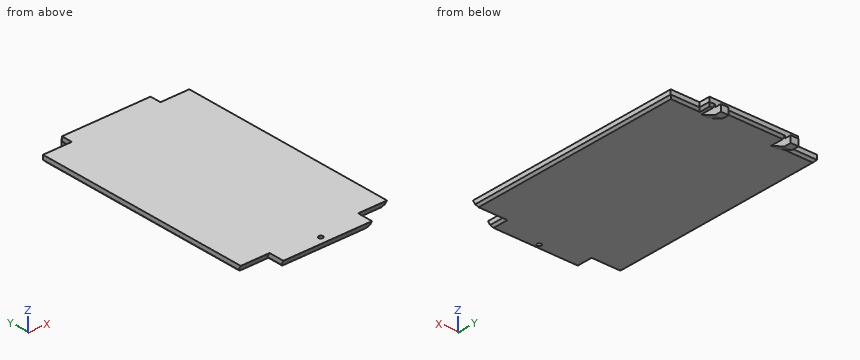
from build123d import *
from OCP.BRepFilletAPI import BRepFilletAPI_MakeChamfer

# Parameters (mm, degrees)
SKETCH_1_W          = 40
SKETCH_1_H          = 112
EXTRUDE_1_DEPTH     = 3
SKETCH_2_R          = 1
CUT_EXTRUDE_1_DEPTH = 3
SKETCH_3_W          = 3.5
SKETCH_3_H          = 10
EXTRUDE_2_DEPTH     = 3.2
CHAMFER_1_SIZE      = 6.8
CHAMFER_1_SIZE2     = 3.170892075
SKETCH_4_W          = 66
SKETCH_4_H          = 100
EXTRUDE_3_DEPTH     = 3
SKETCH_5_W          = 42.259647881
SKETCH_5_H          = 3.16572893
CUT_EXTRUDE_2_DEPTH = 0.2
CHAMFER_3_SIZE      = 1
CHAMFER_4_SIZE      = 2.944486373
CHAMFER_4_SIZE_2    = 1.7


with BuildPart() as part:
    # 草圖1 → 填料-伸長1 (new body)
    with BuildSketch(Plane.XY):
        with Locations((20, 56)):
            Rectangle(SKETCH_1_W, SKETCH_1_H)
    extrude(amount=EXTRUDE_1_DEPTH)

    # 草圖2 → 除料-伸長1 (cut)
    with BuildSketch(Plane.XY):
        with Locations((20, 3.5)):
            Circle(SKETCH_2_R)
    extrude(amount=CUT_EXTRUDE_1_DEPTH, mode=Mode.SUBTRACT)

    # 草圖3 → 填料-伸長2 (add)
    with BuildSketch(Plane.XY):
        with Locations((35.75, 110)):
            Rectangle(SKETCH_3_W, SKETCH_3_H)
        with Locations((4.25, 110)):
            Rectangle(SKETCH_3_W, SKETCH_3_H)
    extrude(amount=-EXTRUDE_2_DEPTH)

    # 導角1: one chamfer whose edges measure the first distance from different faces: ONE call of the kernel's chamfer builder (chamfer() names one face for all edges)
    chamfer_1_edges_1 = [part.edges().sort_by_distance(p)[0] for p in [
        (35.75, 105, -3.2),
    ]]
    chamfer_1_side_1 = [part.faces().sort_by_distance(p)[0] for p in [
        (35.75, 110, -3.2),
    ]]
    chamfer_1_edges_2 = [part.edges().sort_by_distance(p)[0] for p in [
        (4.25, 105, -3.2),
    ]]
    chamfer_1_side_2 = [part.faces().sort_by_distance(p)[0] for p in [
        (4.25, 110, -3.2),
    ]]
    chamfer_1 = BRepFilletAPI_MakeChamfer(part.part.solid().wrapped)
    for e in chamfer_1_edges_1:
        chamfer_1.Add(CHAMFER_1_SIZE, CHAMFER_1_SIZE2, e.wrapped, chamfer_1_side_1[0].wrapped)  # the first distance lies on this face
    for e in chamfer_1_edges_2:
        chamfer_1.Add(CHAMFER_1_SIZE, CHAMFER_1_SIZE2, e.wrapped, chamfer_1_side_2[0].wrapped)  # the first distance lies on this face
    add(Compound.cast(chamfer_1.Shape()), mode=Mode.REPLACE)

    # 草圖4 → 填料-伸長3 (add)
    with BuildSketch(Plane.XY):
        with Locations((20, 57)):
            Rectangle(SKETCH_4_W, SKETCH_4_H)
    extrude(amount=EXTRUDE_3_DEPTH)

    # 草圖5 → 除料-伸長2 (cut)
    with BuildSketch(Plane.XY):
        with Locations((18.12982394, 113.582864465)):
            Rectangle(SKETCH_5_W, SKETCH_5_H)
    extrude(amount=-CUT_EXTRUDE_2_DEPTH, mode=Mode.SUBTRACT)

    # 導角3
    chamfer_3_edges = [part.edges().sort_by_distance(p)[0] for p in [
        (20, 112, 0),
        (1.25, 112, 0),
        (38.75, 112, 0),
        (40, 3.5, 0),
        (0, 109.5, 0),
        (40, 109.5, 0),
        (0, 3.5, 0),
        (-6.5, 107, 0),
        (46.5, 107, 0),
        (53, 57, 0),
        (-13, 57, 0),
    ]]
    chamfer(chamfer_3_edges, length=CHAMFER_3_SIZE)

    # 導角4
    # the kernel refuses this chamfer: 2.944486373, 1.7 mm, written as the material it takes off along each edge
    with BuildSketch(Plane(origin=(8.61763875, 7, 0), x_dir=(0, -0.01932676561270069, 0.9998132206222079), z_dir=(-1, 0, 0))) as chamfer_4_piece_1_section:
        Polygon((CHAMFER_4_SIZE * 0.999813220577, CHAMFER_4_SIZE * 0.0193267656118), (-CHAMFER_4_SIZE_2 * 0.0193267656127, CHAMFER_4_SIZE_2 * 0.999813220622), (0, 0), align=None)
    chamfer_4_piece_1 = extrude(amount=28.2352775, mode=Mode.PRIVATE)
    chamfer_4_piece_1 = split(chamfer_4_piece_1, bisect_by=Plane(origin=(0.556062959, 7.780962214, 0.443937041), z_dir=(-0.7071067811865476, 0, -0.7071067811865476)), keep=Keep.TOP, mode=Mode.PRIVATE)
    chamfer_4_piece_1 = split(chamfer_4_piece_1, bisect_by=Plane(origin=(0, 7.780962214, 0.258582722), z_dir=(1, 0, 0)), keep=Keep.TOP, mode=Mode.PRIVATE)
    add(chamfer_4_piece_1, mode=Mode.SUBTRACT)
    with BuildSketch(Plane(origin=(8.61763875, 7, 0), x_dir=(0, -0.01932676561270069, 0.9998132206222079), z_dir=(-1, 0, 0))) as chamfer_4_piece_2_section:
        Polygon((CHAMFER_4_SIZE * 0.999813220577, CHAMFER_4_SIZE * 0.0193267656118), (-CHAMFER_4_SIZE_2 * 0.0193267656127, CHAMFER_4_SIZE_2 * 0.999813220622), (0, 0), align=None)
    chamfer_4_piece_2 = extrude(amount=28.2352775, mode=Mode.PRIVATE)
    chamfer_4_piece_2 = split(chamfer_4_piece_2, bisect_by=Plane(origin=(-0.79990122, 7.215436489, 1.79990122), z_dir=(0.7071067811865476, 0, 0.7071067811865476)), keep=Keep.TOP, mode=Mode.PRIVATE)
    chamfer_4_piece_2 = split(chamfer_4_piece_2, bisect_by=Plane(origin=(0, 7.215436489, 2.06653496), z_dir=(-1, 0, 0)), keep=Keep.TOP, mode=Mode.PRIVATE)
    add(chamfer_4_piece_2, mode=Mode.SUBTRACT)
    with BuildSketch(Plane(origin=(8.61763875, 7, 0), x_dir=(0, -0.01932676561270069, 0.9998132206222079), z_dir=(-1, 0, 0))) as chamfer_4_piece_3_section:
        Polygon((CHAMFER_4_SIZE * 0.999813220577, CHAMFER_4_SIZE * 0.0193267656118), (-CHAMFER_4_SIZE_2 * 0.0193267656127, CHAMFER_4_SIZE_2 * 0.999813220622), (0, 0), align=None)
    chamfer_4_piece_3 = extrude(amount=28.2352775, mode=Mode.PRIVATE)
    chamfer_4_piece_3 = split(chamfer_4_piece_3, bisect_by=Plane(origin=(-4.964199095, 7.550450485, 5.964199095), z_dir=(-0.7071067811865476, 0, -0.7071067811865476)), keep=Keep.TOP, mode=Mode.PRIVATE)
    chamfer_4_piece_3 = split(chamfer_4_piece_3, bisect_by=Plane(origin=(0, 7.550450485, 0.970145216), z_dir=(-1, 0, 0)), keep=Keep.TOP, mode=Mode.PRIVATE)
    add(chamfer_4_piece_3, mode=Mode.SUBTRACT)
    with BuildSketch(Plane(origin=(59.61763875, 7, 0), x_dir=(0, -0.01932676561270069, 0.9998132206222079), z_dir=(-1, 0, 0))) as chamfer_4_piece_4_section:
        Polygon((CHAMFER_4_SIZE * 0.999813220577, CHAMFER_4_SIZE * 0.0193267656118), (-CHAMFER_4_SIZE_2 * 0.0193267656127, CHAMFER_4_SIZE_2 * 0.999813220622), (0, 0), align=None)
    chamfer_4_piece_4 = extrude(amount=28.2352775, mode=Mode.PRIVATE)
    chamfer_4_piece_4 = split(chamfer_4_piece_4, bisect_by=Plane(origin=(40, 7.550450485, 0.970145216), z_dir=(1, 0, 0)), keep=Keep.TOP, mode=Mode.PRIVATE)
    chamfer_4_piece_4 = split(chamfer_4_piece_4, bisect_by=Plane(origin=(44.964199095, 7.550450485, 5.964199095), z_dir=(0.7071067811865476, 0, -0.7071067811865476)), keep=Keep.TOP, mode=Mode.PRIVATE)
    add(chamfer_4_piece_4, mode=Mode.SUBTRACT)
    with BuildSketch(Plane(origin=(59.61763875, 7, 0), x_dir=(0, -0.01932676561270069, 0.9998132206222079), z_dir=(-1, 0, 0))) as chamfer_4_piece_5_section:
        Polygon((CHAMFER_4_SIZE * 0.999813220577, CHAMFER_4_SIZE * 0.0193267656118), (-CHAMFER_4_SIZE_2 * 0.0193267656127, CHAMFER_4_SIZE_2 * 0.999813220622), (0, 0), align=None)
    chamfer_4_piece_5 = extrude(amount=28.2352775, mode=Mode.PRIVATE)
    chamfer_4_piece_5 = split(chamfer_4_piece_5, bisect_by=Plane(origin=(40, 7.780962214, 0.258582722), z_dir=(-1, 0, 0)), keep=Keep.TOP, mode=Mode.PRIVATE)
    chamfer_4_piece_5 = split(chamfer_4_piece_5, bisect_by=Plane(origin=(39.443937041, 7.780962214, 0.443937041), z_dir=(0.7071067811865476, 0, -0.7071067811865476)), keep=Keep.TOP, mode=Mode.PRIVATE)
    add(chamfer_4_piece_5, mode=Mode.SUBTRACT)
    with BuildSketch(Plane(origin=(59.61763875, 7, 0), x_dir=(0, -0.01932676561270069, 0.9998132206222079), z_dir=(-1, 0, 0))) as chamfer_4_piece_6_section:
        Polygon((CHAMFER_4_SIZE * 0.999813220577, CHAMFER_4_SIZE * 0.0193267656118), (-CHAMFER_4_SIZE_2 * 0.0193267656127, CHAMFER_4_SIZE_2 * 0.999813220622), (0, 0), align=None)
    chamfer_4_piece_6 = extrude(amount=28.2352775, mode=Mode.PRIVATE)
    chamfer_4_piece_6 = split(chamfer_4_piece_6, bisect_by=Plane(origin=(40, 7.215436489, 2.06653496), z_dir=(1, 0, 0)), keep=Keep.TOP, mode=Mode.PRIVATE)
    chamfer_4_piece_6 = split(chamfer_4_piece_6, bisect_by=Plane(origin=(40.79990122, 7.215436489, 1.79990122), z_dir=(-0.7071067811865476, 0, 0.7071067811865476)), keep=Keep.TOP, mode=Mode.PRIVATE)
    add(chamfer_4_piece_6, mode=Mode.SUBTRACT)
    with BuildSketch(Plane(origin=(-6.61763875, 0, 0), x_dir=(0, -0.019326765612700646, 0.9998132206222079), z_dir=(1, 0, 0))) as chamfer_4_piece_7:
        Polygon((CHAMFER_4_SIZE * 0.999813220577, -CHAMFER_4_SIZE * 0.0193267656118), (-CHAMFER_4_SIZE_2 * 0.0193267656127, -CHAMFER_4_SIZE_2 * 0.999813220622), (0, 0), align=None)
    extrude(amount=53.2352775, mode=Mode.SUBTRACT)


solid = part.part
For this review, take the finished solid that the model builds, in its own axes (mm). Give positions to 0.01 mm unless a question says otherwise; leave off trailing zeros. Loops run counter-clockwise (first coordinate to the right, second up) from the corner with the lowest first, then second, coordinate; pieces in that order, holes last. Notation, with made-up numbers: M 73,59.25 L 123,59.25 A12 ccw 123,66.25 Z; hole C 69,69 d1. An arc over 180 degrees is marked long. Answer as a JSON object with one key per item and string values. Group by question number.
Q1. Add section B-B on y = 70. Give the boundary of the cut face in (x, z).
Q2. Add section D-D on x = -3. Give the boundary of the cut face in (y, z), and give its area (3 significant figures).
Q3. Insertion check: P1, Ø2.5, axis at x = 13, z = 1.5, coming from the +Y side; P2, Ø0.9, axis at x = 3.5, y = 113.5, coming from the +Z side; P3, Ø1.6, axis at y = 110, z = 2.5, coming from the -X side; P4, Ø1, axis at x = 41, z = -1, coming from the -Y side. Each pin has a flat end and moves straight along its axis. Give the tip position at first contact, or say it passes through.
Q4. For probe 1 along Z at (x, y) = (18, 80); probe 2 along Y at (x, z) = (20, 1.05); probe 3 along Y at (x, z) = (20, 1.9), list the stretches that pass through material, from the lowest coordinate up. Write a range as [from, to].
Q5. Add section C-C on z = 2. Give the boundary of the cut face in (x, y).
Checked values:
{
 "1": {"outline": "M -13,1 L -12,0 L 52,0 L 53,1 L 53,3 L -13,3 Z"},
 "2": {"outline": "M 7,2.94 L 8.7,0 L 106,0 L 107,1 L 107,3 L 7,3 Z", "area": "297 mm²"},
 "3": {"P1": "y = 112", "P2": "z = -0.2", "P3": "x = 0", "P4": "through"},
 "4": {"probe 1": "[0, 3]", "probe 2": "[1.09, 2.5], [4.5, 112]", "probe 3": "[0.6, 2.5], [4.5, 112]"},
 "5": {"outline": "M -13,7.55 L 0,7.55 L 0,0.55 L 40,0.55 L 40,7.55 L 53,7.55 L 53,107 L 40,107 L 40,112 L 0,112 L 0,107 L -13,107 Z; hole C 20,3.5 d2"}
}
